from build123d import *

# Parameters (mm, degrees)
F0_R     = 25.4
F1_DEPTH = 69.85
F2_R     = 12.7
F3_R     = 12.6922098365
F4_DEPTH = 43.18
F5_R     = 5.08
F6_R     = 2.54


with BuildPart() as f1:
    # F0 (on Top) → F1 (new body, symmetric)
    with BuildSketch(Plane.XY):
        Circle(F0_R)
    extrude(amount=F1_DEPTH, both=True)

    # F2
    f2_edges = [f1.edges().sort_by_distance(p)[0] for p in [
        (-25.4, 0, 69.85),
    ]]
    fillet(f2_edges, radius=F2_R)

    # F3 (on face) → F4 (join)
    with BuildSketch(Plane.XY.offset(69.85)):
        Circle(F3_R)
    extrude(amount=F4_DEPTH)

    # F5
    f5_edges = [f1.edges().sort_by_distance(p)[0] for p in [
        (-12.69221, 0, 113.03),
    ]]
    fillet(f5_edges, radius=F5_R)

    # F6
    f6_edges = [f1.edges().sort_by_distance(p)[0] for p in [
        (-12.7, 0, 69.85),
        (-12.69221, 0, 69.85),
    ]]
    fillet(f6_edges, radius=F6_R)


solid = f1.part
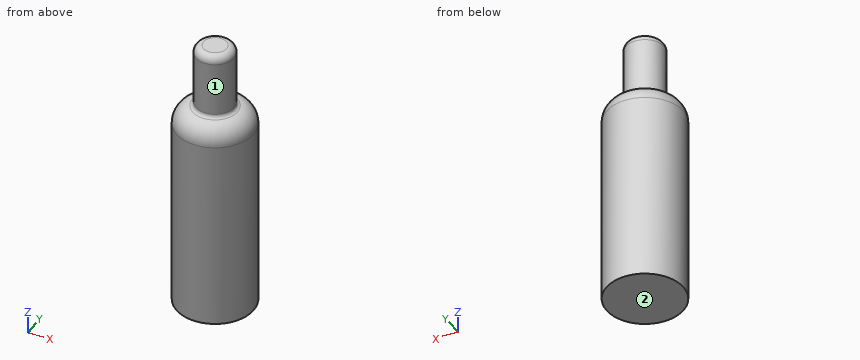
Verification items for the finished model (mm, model axes). Face numbers are marked on the shaded views. A direction names the side the tool comes from. Coordinates: 2 decimals unless noted, no trailing zeros. Write each loop counter-clockwise with the first axis right and the second up, starting at its lowest first coordinate (ties: lowest second). Pieces come first, ordered by that corner, then holes. Notation, with made-up numbers: (-19, 43) - (29, 43) arc R3 cw to (29, 47) - close; hole circle Ø10 at (81.25, -3). An arc over 180 degrees is marked (long way). Answer as a JSON object with one key per item and string values.
(1) Gauge pin test, flat ends, axial feed: pin 1 Ø1.5 at (y, z) = (-19.5, 10) entering from +X; pin 2 Ø5 at (y, z) = (-13, -27.5) entering from +X; pin 3 Ø1 at (x, z) = (20, -30.5) entering from -Y. Record the tip position at first contact, or that the pin passes through.
Report:
{"pin 1": "x = 17.13", "pin 2": "x = 23.13", "pin 3": "y = -16.28"}
(2) Tool access check on the marked faces 1 and 2. Record the directions out of +Z, -Z, +X, -X, +Y, -Y that give a thin tool (end or side, any length) a straight path to the whole face; none if there is none.
Report:
{"face 1": "+Z", "face 2": "-Z, +X, -X, +Y, -Y"}
(3) Cross-section at A-A on z = 36. Record the cut outline in (x, y).
Report:
{"outline": "circle Ø50.8 at (0, 0)"}
(4) Thickness scan on line 1 along Z through (x, y) = (-8, 12.5); line 2 along Y through (x, z) = (-0.5, -16.5); line 3 along X through (y, z) = (11, 105.5). Record the ranges inside material, lowest first.
Report:
{"line 1": "-69.85 to 69.67", "line 2": "-25.4 to 25.4", "line 3": "-6.33 to 6.33"}
